The listing builds one solid part. Answer for the finished solid, in the listing's coordinates (mm). A direction names the side the tool comes from. Coordinates: 2 decimals unless noted, no trailing zeros. Write each loop counter-clockwise with the first axis right and the second up, starting at its lowest first coordinate (ties: lowest second). Pieces come first, ordered by that corner, then holes.
```python
from build123d import *

# Parameters (mm, degrees)
BOSS_EXTRUDE1_DEPTH      = 10
BOSS_EXTRUDE1_DEPTH_BACK = 10
SKETCH1_W                = 40
SKETCH1_H                = 40
SKETCH2_W                = 10
SKETCH2_H                = 10
CUT_EXTRUDE1_DEPTH       = 5


with BuildPart() as part:
    # Sketch1 → Boss-Extrude1 (new, two sides: drawn at the far end of the back side and taken through both)
    with BuildSketch(Plane.XY.offset(-BOSS_EXTRUDE1_DEPTH_BACK)):
        with Locations((20, 20)):
            Rectangle(SKETCH1_W, SKETCH1_H)
    extrude(amount=BOSS_EXTRUDE1_DEPTH + BOSS_EXTRUDE1_DEPTH_BACK)

    # Sketch2 → Cut-Extrude1 (cut)
    with BuildSketch(Plane.XY):
        with Locations((5, 5)):
            Rectangle(SKETCH2_W, SKETCH2_H)
    extrude(amount=CUT_EXTRUDE1_DEPTH, mode=Mode.SUBTRACT)


solid = part.part
```
(1) Find the intervals of material crossed by probe 1 along Z at (x, y) = (3.5, 2); probe 2 along Y at (x, z) = (6, 3.75), in increasing order.
(2) For a pull along Z with two mould halves and no side action, classify faces 3 (the flat face through (20, 40, 0)), 4 (the flat face through (20, 20, -10)), 5 (the flat face through (5, 5, 0)) as pulls with the +Z half, pulls with the -Z half, needs draft (parallel to the pull), parting line crosses it, or undercut.
(3) Section A-A, the plane y = 8 is taken. Write down the section's boundary in (x, z), plus the area to 3 significant figures.
(4) Section C-C, the plane z = 4 is taken. Write down the section's boundary in (x, y), plus the area to 3 significant figures.
(5) Each of these flat-tipped pins is pushed along its axis until it touches: pin 1 (2.5 mm diameter, centred on x = 6.5, z = 2, fed in from -Y); pin 2 (8 mm diameter, centred on y = 8.5, z = 7.5, fed in from -X); pin 3 (2.5 mm diameter, centred on y = 6.5, z = 3.5, fed in from -X). Where does it stop, or does it pass through?
(6) Which of the six approach directions +Z, -Z, +X, -X, +Y, -Y give full straight-line access (tool end or side, diameter ignored) to faces 1 (the flat face through (40, 20, 0)), 2 (the flat face through (10, 5, 2))?
Solution:
1. probe 1: z = -10 to 0, 5 to 10
1. probe 2: y = 10 to 40
2. face 3: needs draft
2. face 4: pulls with the -Z half
2. face 5: undercut
3. outline: (0, -10) - (40, -10) - (40, 10) - (0, 10) - (0, 5) - (10, 5) - (10, 0) - (0, 0) - close
3. area: 750 mm2
4. outline: (0, 10) - (10, 10) - (10, 0) - (40, 0) - (40, 40) - (0, 40) - close
4. area: 1,500 mm2
5. pin 1: stops at y = 10
5. pin 2: stops at x = 0
5. pin 3: stops at x = 10
6. face 1: +Z, -Z, +X, +Y, -Y
6. face 2: -X, -Y
